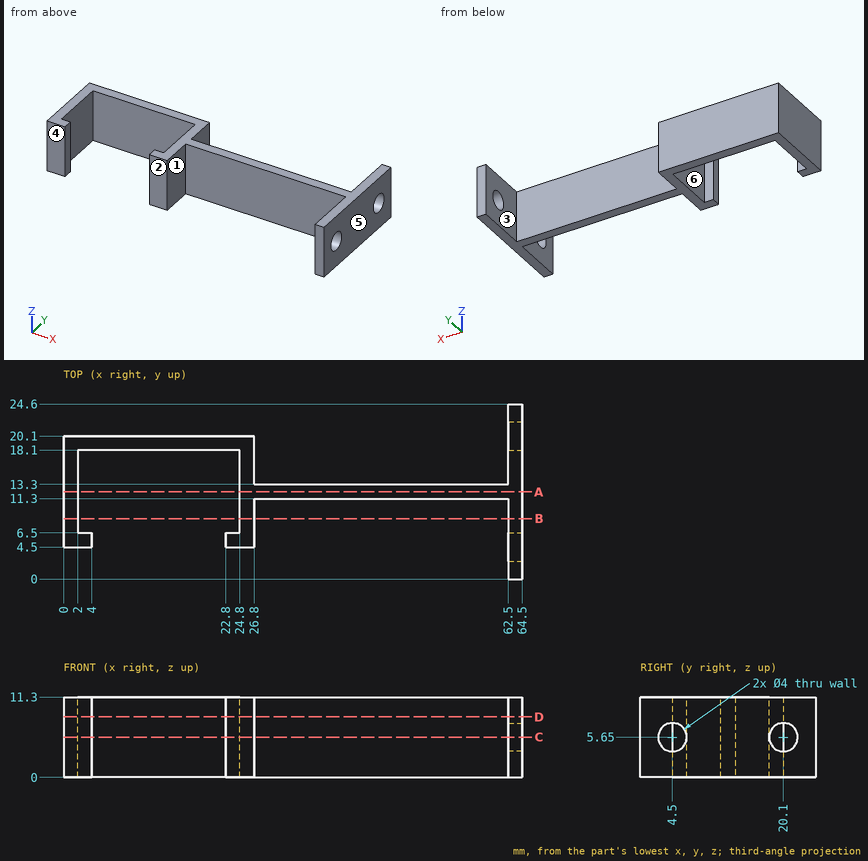
Geometry check sheet. Reference: drawing and pictorial views, mm from the part's lowest x, y, z. A direction names the side the tool comes from. Give positions to 0.01 mm unless a question says otherwise; leave off trailing zeros. Write each loop counter-clockwise with the first axis right and the second up, starting at its lowest first coordinate (ties: lowest second). Pieces come first, ordered by that corner, then holes. Notation, with made-up numbers: M -24,68 L -14,68 A20 cw -14,95 Z; hole C 18.5,-10.5 d4. An arc over 180 degrees is marked long. Put each result on its own line as item: value. Start each with the question number.
1. Section check B-B (y = 8.5). Record the cut outline in (x, z), and give its area (3 significant figures).
2. Scan lines: line 1 along X through (y, z) = (17.5, 7.25); line 2 along Y through (x, z) = (63.3, 5.65); line 3 along X through (y, z) = (12.75, 1.25). Record each from-to range of solid material in increasing order. Write a range as [from, to].
3. Draft check along X on the marked faces 4, 5 and 6. Enter one of: +X half, -X half, draft (parallel to the pull), parting line (faces both ways), or undercut.
4. Set-up check for the marked faces 1, 2 and 3: record each of +Z, -Z, +X, -X, +Y, -Y from which the full face is reachable in a straight line by a thin tool's end or side.
5. Go/stop test with flat-tipped pins: pin 1 Ø2 at (x, z) = (22, 1.5) entering from +Y; pin 2 Ø3 at (x, z) = (2, 6.5) entering from -Y; pin 3 Ø5 at (x, z) = (46.5, 3.5) entering from +Y. Record where each tip stops, or that it passes through.
6. Section check C-C (z = 5.65). Record the cut outline in (x, y).
7. Section check D-D (z = 8.5). Record the cut outline in (x, y), and give its area (3 significant figures).
8. Section check A-A (y = 12.25). Record the cut outline in (x, z), and give its area (3 significant figures).
Answer list:
1. outline: M 0,0 L 2,0 L 2,11.3 L 0,11.3 Z; M 24.8,0 L 26.8,0 L 26.8,11.3 L 24.8,11.3 Z; M 62.5,0 L 64.5,0 L 64.5,11.3 L 62.5,11.3 Z
1. area: 67.8 mm2
2. line 1: [0, 2], [24.8, 26.8], [62.5, 64.5]
2. line 2: [0, 2.5], [6.5, 18.1], [22.1, 24.6]
2. line 3: [0, 2], [24.8, 64.5]
3. face 4: draft
3. face 5: +X half
3. face 6: undercut
4. face 1: +Z, -Z, -Y
4. face 2: +Z, -Z, -X, -Y
4. face 3: +Z, -Z, +Y
5. pin 1: y = 20.1
5. pin 2: y = 4.5
5. pin 3: y = 13.3
6. outline: M 0,4.5 L 4,4.5 L 4,6.5 L 2,6.5 L 2,18.1 L 24.8,18.1 L 24.8,6.5 L 22.8,6.5 L 22.8,4.5 L 26.8,4.5 L 26.8,11.3 L 62.5,11.3 L 62.5,6.5 L 64.5,6.5 L 64.5,18.1 L 62.5,18.1 L 62.5,13.3 L 26.8,13.3 L 26.8,20.1 L 0,20.1 Z; M 62.5,0 L 64.5,0 L 64.5,2.5 L 62.5,2.5 Z; M 62.5,22.1 L 64.5,22.1 L 64.5,24.6 L 62.5,24.6 Z
7. outline: M 0,4.5 L 4,4.5 L 4,6.5 L 2,6.5 L 2,18.1 L 24.8,18.1 L 24.8,6.5 L 22.8,6.5 L 22.8,4.5 L 26.8,4.5 L 26.8,11.3 L 62.5,11.3 L 62.5,0 L 64.5,0 L 64.5,24.6 L 62.5,24.6 L 62.5,13.3 L 26.8,13.3 L 26.8,20.1 L 0,20.1 Z
7. area: 237 mm2
8. outline: M 0,0 L 2,0 L 2,11.3 L 0,11.3 Z; M 24.8,0 L 64.5,0 L 64.5,11.3 L 24.8,11.3 Z
8. area: 471 mm2
